Model file for the job. Use its own axes, mm. Face numbers are marked on the shaded views. A direction names the side the tool comes from. Coordinates: 2 decimals unless noted, no trailing zeros. Loops run counter-clockwise (first coordinate to the right, second up) from the corner with the lowest first, then second, coordinate; pieces in that order, holes last. Notation, with made-up numbers: (84.5, 12) -> (88.5, 12) arc R23 cw to (88.5, 30) -> close; hole circle Ø10 at (-3, 83). An arc over 180 degrees is marked (long way). Use one line per item in the form item = value.
```python
from build123d import *

# Parameters (mm, degrees)
F1_DEPTH = 19.4
F0_R     = 2.1
F2_DEPTH = 0.9
F3_DEPTH = 1.25
F4_DEPTH = 3.29
F5_DEPTH = 9.4


with BuildPart() as f1:
    # F0 (on Front) → F1 (new body)
    with BuildSketch(Plane.XZ):
        with BuildLine():
            ThreePointArc((-13.7181048254, 3.55), (-14.17, 0), (-13.7181048254, -3.55))
            Line((-13.7181048254, -3.55), (13.7181048254, -3.55))
            ThreePointArc((13.7181048254, -3.55), (14.056572224, -1.7893231436), (14.17, 0))
            ThreePointArc((14.17, 0), (14.056572224, 1.7893231436), (13.7181048254, 3.55))
            Line((13.7181048254, 3.55), (1.0858637115, 3.55))
            ThreePointArc((1.0858637115, 3.55), (0, 3.42), (-1.0858637115, 3.55))
            Line((-1.0858637115, 3.55), (-13.7181048254, 3.55))
        make_face()
        with BuildLine():
            ThreePointArc((13.7181048254, 3.55), (0, 14.17), (-13.7181048254, 3.55))
            Line((-13.7181048254, 3.55), (-1.0858637115, 3.55))
            ThreePointArc((-1.0858637115, 3.55), (-2.842976163, 11.6362807602), (4.6, 8.02))
            ThreePointArc((4.6, 8.02), (3.6162807602, 5.177023837), (1.0858637115, 3.55))
            Line((1.0858637115, 3.55), (13.7181048254, 3.55))
        make_face()
        with BuildLine():
            ThreePointArc((-13.7181048254, -3.55), (-11.8586491349, -7.7563741977), (-8.75, -11.1456897499))
            Line((-8.75, -11.1456897499), (8.75, -11.1456897499))
            ThreePointArc((8.75, -11.1456897499), (11.8586491349, -7.7563741977), (13.7181048254, -3.55))
            Line((13.7181048254, -3.55), (-13.7181048254, -3.55))
        make_face()
        with BuildLine():
            ThreePointArc((8.75, -11.1456897499), (0, -14.17), (-8.75, -11.1456897499))
            Line((-8.75, -11.1456897499), (-8.75, -16.9456897499))
            Line((-8.75, -16.9456897499), (8.75, -16.9456897499))
            Line((8.75, -16.9456897499), (8.75, -11.1456897499))
        make_face()
        with BuildLine():
            Line((8.75, -11.1456897499), (-8.75, -11.1456897499))
            ThreePointArc((-8.75, -11.1456897499), (0, -14.17), (8.75, -11.1456897499))
        make_face()
        with BuildLine():
            ThreePointArc((4.6, 8.02), (-2.842976163, 11.6362807602), (-1.0858637115, 3.55))
            Line((-1.0858637115, 3.55), (1.0858637115, 3.55))
            ThreePointArc((1.0858637115, 3.55), (3.6162807602, 5.177023837), (4.6, 8.02))
        make_face()
        with BuildLine():
            ThreePointArc((1.475, 10.0385081124), (2.2290693125, 9.1519231423), (2.5, 8.02))
            ThreePointArc((2.5, 8.02), (2.2290693125, 6.8880768577), (1.475, 6.0014918876))
            ThreePointArc((1.475, 6.0014918876), (0, 5.52), (-1.475, 6.0014918876))
            ThreePointArc((-1.475, 6.0014918876), (-2.5, 8.02), (-1.475, 10.0385081124))
            ThreePointArc((-1.475, 10.0385081124), (0, 10.52), (1.475, 10.0385081124))
        make_face(mode=Mode.SUBTRACT)
        with BuildLine():
            Line((1.475, 6.0014918876), (1.475, 10.0385081124))
            ThreePointArc((1.475, 10.0385081124), (0, 10.52), (-1.475, 10.0385081124))
            Line((-1.475, 10.0385081124), (-1.475, 6.0014918876))
            ThreePointArc((-1.475, 6.0014918876), (0, 5.52), (1.475, 6.0014918876))
        make_face()
        with BuildLine():
            ThreePointArc((1.475, 6.0014918876), (2.2290693125, 6.8880768577), (2.5, 8.02))
            ThreePointArc((2.5, 8.02), (2.2290693125, 9.1519231423), (1.475, 10.0385081124))
            Line((1.475, 10.0385081124), (1.475, 6.0014918876))
        make_face()
        with BuildLine():
            Line((-1.475, 6.0014918876), (-1.475, 10.0385081124))
            ThreePointArc((-1.475, 10.0385081124), (-2.5, 8.02), (-1.475, 6.0014918876))
        make_face()
    extrude(amount=F1_DEPTH)

    # F0 (on Front) → F2 (join)
    with BuildSketch(Plane.XZ):
        with BuildLine():
            ThreePointArc((14.17, 0), (14.056572224, -1.7893231436), (13.7181048254, -3.55))
            Line((13.7181048254, -3.55), (17.45, -3.55))
            ThreePointArc((17.45, -3.55), (19.9602290732, -2.5102290732), (21, 0))
            ThreePointArc((21, 0), (19.9602290732, 2.5102290732), (17.45, 3.55))
            Line((17.45, 3.55), (13.7181048254, 3.55))
            ThreePointArc((13.7181048254, 3.55), (14.056572224, 1.7893231436), (14.17, 0))
        make_face()
        with Locations((18.0333442986, 0)):
            Circle(F0_R, mode=Mode.SUBTRACT)
        with BuildLine():
            Line((-17.45, -3.55), (-13.7181048254, -3.55))
            ThreePointArc((-13.7181048254, -3.55), (-14.17, 0), (-13.7181048254, 3.55))
            Line((-13.7181048254, 3.55), (-17.45, 3.55))
            ThreePointArc((-17.45, 3.55), (-19.9602290732, 2.5102290732), (-21, 0))
            ThreePointArc((-21, 0), (-19.9602290732, -2.5102290732), (-17.45, -3.55))
        make_face()
        with Locations((-18.0333442986, 0)):
            Circle(F0_R, mode=Mode.SUBTRACT)
    extrude(amount=F2_DEPTH)

    # F0 (on Front) → F3 (join)
    with BuildSketch(Plane.XZ):
        with BuildLine():
            ThreePointArc((4.6, 8.02), (-2.842976163, 11.6362807602), (-1.0858637115, 3.55))
            Line((-1.0858637115, 3.55), (1.0858637115, 3.55))
            ThreePointArc((1.0858637115, 3.55), (3.6162807602, 5.177023837), (4.6, 8.02))
        make_face()
        with BuildLine():
            ThreePointArc((1.475, 10.0385081124), (2.2290693125, 9.1519231423), (2.5, 8.02))
            ThreePointArc((2.5, 8.02), (2.2290693125, 6.8880768577), (1.475, 6.0014918876))
            ThreePointArc((1.475, 6.0014918876), (0, 5.52), (-1.475, 6.0014918876))
            ThreePointArc((-1.475, 6.0014918876), (-2.5, 8.02), (-1.475, 10.0385081124))
            ThreePointArc((-1.475, 10.0385081124), (0, 10.52), (1.475, 10.0385081124))
        make_face(mode=Mode.SUBTRACT)
    extrude(amount=-F3_DEPTH)

    # F0 (on Front) → F4 (join)
    with BuildSketch(Plane.XZ):
        with BuildLine():
            Line((-1.475, 6.0014918876), (-1.475, 10.0385081124))
            ThreePointArc((-1.475, 10.0385081124), (-2.5, 8.02), (-1.475, 6.0014918876))
        make_face()
        with BuildLine():
            Line((1.475, 6.0014918876), (1.475, 10.0385081124))
            ThreePointArc((1.475, 10.0385081124), (0, 10.52), (-1.475, 10.0385081124))
            Line((-1.475, 10.0385081124), (-1.475, 6.0014918876))
            ThreePointArc((-1.475, 6.0014918876), (0, 5.52), (1.475, 6.0014918876))
        make_face()
        with BuildLine():
            ThreePointArc((1.475, 6.0014918876), (2.2290693125, 6.8880768577), (2.5, 8.02))
            ThreePointArc((2.5, 8.02), (2.2290693125, 9.1519231423), (1.475, 10.0385081124))
            Line((1.475, 10.0385081124), (1.475, 6.0014918876))
        make_face()
    extrude(amount=-F4_DEPTH)

    # F0 (on Front) → F5 (join)
    with BuildSketch(Plane.XZ):
        with BuildLine():
            Line((1.475, 6.0014918876), (1.475, 10.0385081124))
            ThreePointArc((1.475, 10.0385081124), (0, 10.52), (-1.475, 10.0385081124))
            Line((-1.475, 10.0385081124), (-1.475, 6.0014918876))
            ThreePointArc((-1.475, 6.0014918876), (0, 5.52), (1.475, 6.0014918876))
        make_face()
    extrude(amount=-F5_DEPTH)


solid = f1.part
```
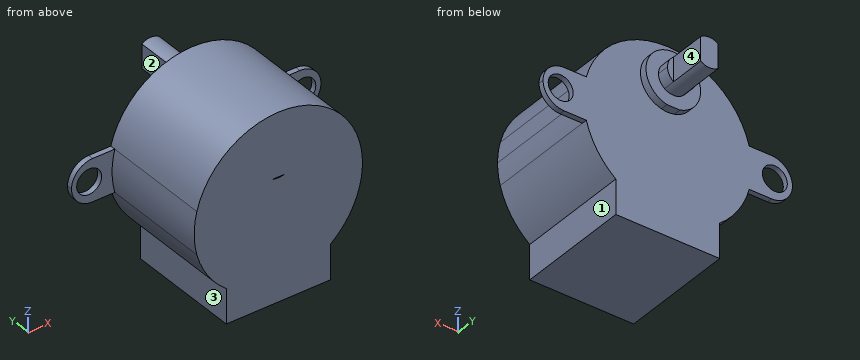
Q1. Band-saw the part on B-B, the plane y = -6. Write the cut outline in (x, z).
Result:
outline = (-8.75, -16.95) -> (8.75, -16.95) -> (8.75, -11.15) arc R14.17 ccw (long way) to (-8.75, -11.15) -> close; hole (-1.09, 3.55) arc R4.6 ccw to (1.09, 3.55) -> close
Q2. Wall check: line 1 along Y through (x, z) = (-3.5, -4); line 2 along Z through (x, y) = (3.5, -17); line 3 along X through (y, z) = (-5.75, -14.5). Give the ranges that are in metal, low to high.
Result:
line_1 = -19.4 to 0
line_2 = -16.95 to 13.73
line_3 = -8.75 to 8.75
Q3. Which spindle directions (+Z, -Z, +X, -X, +Y, -Y) get a long thin tool onto all of the face, cutting with end or side? Do the marked faces 1, 2, 3 and 4. Say none if no direction does.
Result:
face_1 = -Z, +X, +Y, -Y
face_2 = +Z, -Z, -X, +Y
face_3 = -Z, -X, +Y, -Y
face_4 = +Z, -Z, +X, +Y
Q4. Band-saw the part on A-A, the plane x = 0. Write the cut outline in (y, z).
Result:
outline = (-19.4, -16.95) -> (0, -16.95) -> (0, 3.42) -> (-19.4, 3.42) -> close; (-19.4, 3.55) -> (1.25, 3.55) -> (1.25, 5.52) -> (9.4, 5.52) -> (9.4, 10.52) -> (1.25, 10.52) -> (1.25, 12.62) -> (0, 12.62) -> (0, 14.17) -> (-19.4, 14.17) -> close
Q5. Band-saw the part on C-C, the plane z = -15. Write the cut outline in (x, y), and give its area (4 significant figures).
Result:
outline = (-8.75, -19.4) -> (8.75, -19.4) -> (8.75, 0) -> (-8.75, 0) -> close
area = 339.5 mm2
Q6. Pin check, flat tips, straight feed: pin 1 Ø6.5 at (y, z) = (-11.5, -14) entering from +X; pin 2 Ø10 at (x, z) = (-2.5, -6.5) entering from +Y; pin 3 Ø0.8 at (x, z) = (2, 8.5) entering from +Y. Stop position of each tip, or through.
Result:
pin_1 = 9.23
pin_2 = 0
pin_3 = 3.29
Q7. Band-saw the part on D-D, the plane x = 12. Write the cut outline in (y, z), and give its area (3 significant figures).
Result:
outline = (-19.4, -7.54) -> (0, -7.54) -> (0, 7.54) -> (-19.4, 7.54) -> close
area = 292 mm2
